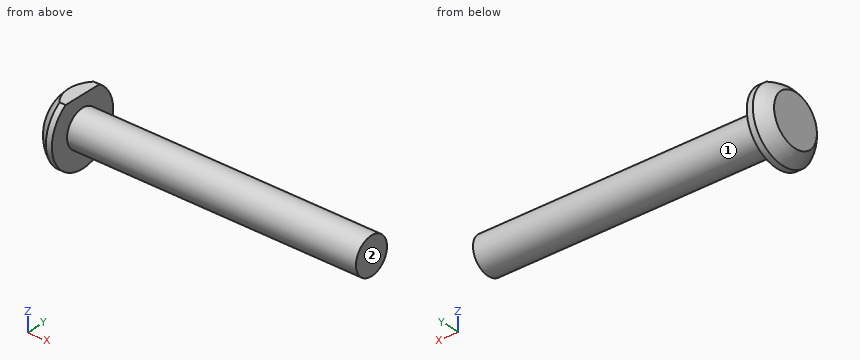
```python
from build123d import *

# Parameters (mm, degrees)
F0_W     = 76.2
F0_H     = 4.826
F2_W     = 10.530284
F2_H     = 4.986605
F3_DEPTH = 25.4


with BuildPart() as f1:
    # F0 (on Front) → F1 (revolve)
    with BuildSketch(Plane.XZ):
        Polygon((-422.80503, 234.378874), (-422.80503, 239.204874), (-422.80503, 243.903874), (-424.39253, 243.903874), (-424.39253, 234.378874), align=None)
        with Locations((-384.70503, 236.791874)):
            Rectangle(F0_W, F0_H)
        with BuildLine():
            Line((-424.39253, 234.378874), (-424.39253, 243.903874))
            ThreePointArc((-424.39253, 243.903874), (-426.119453, 242.623521), (-427.56753, 241.034608))
            Line((-427.56753, 241.034608), (-427.56753, 234.378874))
            Line((-427.56753, 234.378874), (-424.39253, 234.378874))
        make_face()
    revolve(axis=Axis((-387.08628, 0, 234.378874), (1, 0, 0)))

    # F2 (on face) → F3 (cut)
    with BuildSketch(Plane.YZ.offset(-422.80503)):
        with Locations((0, 244.809676)):
            Rectangle(F2_W, F2_H)
    extrude(amount=-F3_DEPTH, mode=Mode.SUBTRACT)


solid = f1.part
```
Design review of the part built by this model. Coordinates are the model's own, in mm. Face numbers are marked on the shaded views. A direction names the side the tool comes from. Give positions to 0.01 mm unless a question says otherwise; leave off trailing zeros. Order: outer loops, then holes, each group sorted by start corner. A loop starts at its lowest first (then second) coordinate and runs counter-clockwise, first axis right, second up. Notation, with made-up numbers: (64.25, 63) -> (82.25, 63) arc R13 ccw to (82.25, 71) -> close; hole circle Ø8 at (82, 18). An arc over 180 degrees is marked (long way). Write item = value, one per line. Start each with the question number.
(1) To check wall thickness, follow line 1 along X through (y, z) = (3.75, 238.25); line 2 along Y through (x, z) = (-355.5, 232); line 3 along Z through (x, y) = (-358, -0.25). State the ranges of each line that lie inside material, in increasing order.
(2) We need section A-A on x = -372. Write out the cut boundary in (y, z).
(3) For the marked faces 1 and 2, list the 3-axis set-ups (+Z, -Z, +X, -X, +Y, -Y) from which the entire face can be reached by the end or side of a thin tool; tool diameter is ignored.
(4) For pin 1 (5 mm diameter, centred on x = -368, y = -4, fed in from -Z); pin 2 (6 mm diameter, centred on x = -372.5, z = 236, fed in from -Y); pin 3 (4 mm diameter, centred on x = -402.5, y = 3.5, fed in from +Z); pin 4 (5 mm diameter, centred on y = 1.5, z = 227, fed in from -X), all flat-tipped, find the tip position at first contact; note any pin that passes through.
Numbers:
q1.line_1 = -427.57 to -422.81
q1.line_2 = -4.2 to 4.2
q1.line_3 = 229.56 to 239.2
q2.outline = circle Ø9.65 at (0, 234.38)
q3.face_1 = +X
q3.face_2 = +Z, -Z, +X, +Y, -Y
q4.pin_1 = 229.79
q4.pin_2 = -4.83
q4.pin_3 = 238.97
q4.pin_4 = -427.57
